Autodesk Inventor part; units mm, degrees
ref_plane "YZ Plane" through (0, 0, 0) normal (1, 0, 0) x (0, 1, 0)
ref_plane "XZ Plane" through (0, 0, 0) normal (0, 1, 0) x (-1, 0, 0)
ref_plane "XY Plane" through (0, 0, 0) normal (0, 0, 1) x (1, 0, 0)
sketch "Sketch1" plane through (0, 0, 0) normal (0, 0, 1) x (1, 0, 0)
  line L0 (-240, -100) -> (240, -100)
  line L1 (240, -100) -> (240, 100)
  line L2 (240, 100) -> (-240, 100)
  line L3 (-240, 100) -> (-240, -100)
  line L4 (-240, -100) -> (240, 100) construction
  line L5 (240, -100) -> (-240, 100) construction
  point P0 (0, 0)
  dimension "d0" = 480
  dimension "d1" = 200
extrude "Plate1" add sketch "Sketch1" along normal blind 2
sketch "Sketch2" plane through (0, 0, 0) normal (0, 0, -1) x (-1, 0, 0)
  line L0 (-220, 80) -> (-20, 80) construction
  line L1 (-20, 80) -> (-20, 60) construction
  line L2 (-20, 60) -> (-220, 60) construction
  line L3 (-220, 60) -> (-220, 80) construction
  line L4 (-240, 100) -> (240, 100)
  line L5 (-240, -100) -> (-240, 100)
  point P0 (0, 0)
  dimension "d6" = 200
  dimension "d9" = 20
  dimension "d10" = 20
  dimension "d11" = 20
mark "Mark1"
sketch "Sketch3" plane through (240, -98, 0) normal (0, -1, 0) x (1, 0, 0)
  line L0 (-480, 0) -> (0, 0)
  line L1 (0, 0) -> (0, 30)
  line L2 (0, 30) -> (-480, 30)
  line L3 (-480, 30) -> (-480, 0)
edge flange "Flange1" height 30 angle 90 thickness 2 bend radius 2.75 thickness toward (0, -1, 0) relief round relief width 2 relief depth 1 edges at (0, -100, 2) wall of the first edge with corners at (-240, -98, 0) (240, -98, 0) (240, -98, 30) (-240, -98, 30)
bend "Bend1"
corner "Corner1"
sketch "Sketch4" plane through (-240, -98, 30) normal (0, 1, 0) x (1, 0, 0)
  line L0 (480, 25.25) -> (0, 25.25)
  line L1 (0, 25.25) -> (0, 0)
  line L2 (0, 0) -> (480, 0)
  line L3 (480, 25.25) -> (480, 0)
  circle A0 centre (240, 10) radius 5
  point P0 (240, 30)
  point P1 (240, 25.25)
  point P2 (240, 0)
  dimension "d22" = 10
  dimension "d23" = 10
extrude "Cut1" cut sketch "Sketch4" against normal blind 2 contours A0
pattern_linear "Rectangular Pattern1" count 3 spacing 200 along (1, 0, 0) of "Cut1" first direction both ways yes
equation "\"d24\" = Thickness"
equation "\"d2\" = Thickness"
equation "\"d12\" = BendReliefWidth"
equation "\"d13\" = BendReliefDepth"
equation "\"d14\" = MinimumRemnant"
equation "\"d15\" = TransitionRadius"
equation "\"d18\" = BendRadius"
equation "\"d19\" = CornerReliefSize"
equation "\"d20\" = GapSize"
equation "\"d21\" = JacobiRadiusSize"
equation "\"BendReliefWidth\" = Thickness"
equation "\"BendReliefDepth\" = 0.5 * Thickness"
equation "\"CornerReliefSize\" = 4 * Thickness"
equation "\"MinimumRemnant\" = 2 * Thickness"
equation "\"TransitionRadius\" = BendRadius"
equation "\"JacobiRadiusSize\" = BendRadius"
equation "\"GapSize\" = Thickness"
properties part number "TRM 014 face main" material "AISI 304"
Read the model definition and answer for the solid it produces. Units are mm, in the model's axes. A direction names the side the tool comes from. Give positions to 0.01 mm unless a question says otherwise; leave off trailing zeros. Write each loop counter-clockwise with the first axis right and the second up, starting at its lowest first coordinate (ties: lowest second). Pieces come first, ordered by that corner, then holes. Notation, with made-up numbers: (17, 20) -> (55, 20) arc R25 ccw to (55, 34) -> close; hole circle Ø9 at (32.5, 65). An arc over 180 degrees is marked (long way). Answer as a JSON object with one key per item and string values.
1) Section D-D on y = 15 is taken. Write down the section's boundary in (x, z), then the cut area to 3 significant figures.
Findings below:
{"outline": "(-240, 0) -> (240, 0) -> (240, 2) -> (-240, 2) -> close", "area": "960 mm^2"}
2) For a pull along Z with two mould halves and no side action, classify faces 1 (the flat face through (-3, 4, 2)), 2 (the cylindrical face through (202.307, -98.986, 24.436)), 3 (the flat face through (3, -100, 15)) as pulls with the +Z half, pulls with the -Z half, needs draft (parallel to the pull), parting line crosses it, or undercut.
Findings below:
{"face 1": "pulls with the +Z half", "face 2": "undercut", "face 3": "needs draft"}
3) Straight lines are drawn through the part: probe 1 along X at (y, z) = (-98.7, 20); probe 2 along Z at (x, y) = (200, -99.05); probe 3 along Y at (x, z) = (203, 27.5). For each, find the intervals that lie inside material, in ascending order. Write a range as from..to.
Findings below:
{"probe 1": "x = -240..-205, -195..-5, 5..195, 205..240", "probe 2": "z = 1.9..15, 25..30", "probe 3": "y = -100..-98"}
4) Section B-B on z = 20 is taken. Write down the section's boundary in (x, y).
Findings below:
{"outline": "(-240, -100) -> (-205, -100) -> (-205, -98) -> (-240, -98) -> close; (-195, -100) -> (-5, -100) -> (-5, -98) -> (-195, -98) -> close; (5, -100) -> (195, -100) -> (195, -98) -> (5, -98) -> close; (205, -100) -> (240, -100) -> (240, -98) -> (205, -98) -> close"}
5) Flat-ended cylindrical pins translate along their axes: pin 1 Ø12 at (x, y) = (-95, -57) entering from -Z; pin 2 Ø1 at (x, z) = (180.5, 24) entering from +Y; pin 3 Ø8 at (x, z) = (0, 20) entering from -Y. Find the tip coordinate at first contact, or state that the pin passes through.
Findings below:
{"pin 1": "stops at z = 0", "pin 2": "stops at y = -98", "pin 3": "passes through"}
6) Section A-A on x = -200 is taken. Write down the section's boundary in (y, z), then the cut area to 3 significant figures.
Findings below:
{"outline": "(-100, 4.75) arc R4.75 ccw to (-95.25, 0) -> (100, 0) -> (100, 2) -> (-95.25, 2) arc R2.75 cw to (-98, 4.75) -> (-98, 15) -> (-100, 15) -> close; (-100, 25) -> (-98, 25) -> (-98, 30) -> (-100, 30) -> close", "area": "433 mm^2"}
7) Section C-C on x = -29.5 is taken. Write down the section's boundary in (y, z).
Findings below:
{"outline": "(-100, 4.75) arc R4.75 ccw to (-95.25, 0) -> (100, 0) -> (100, 2) -> (-95.25, 2) arc R2.75 cw to (-98, 4.75) -> (-98, 30) -> (-100, 30) -> close"}
8) A tool of negligible diameter and unlimited length cuts with its end or side. For faces 4 (the flat face through (3, -98, 14)), 5 (the cylindrical face through (-197.693, -98.986, 24.436)), from which of +Z, -Z, +X, -X, +Y, -Y can it reach the whole face along a straight path? Write none if from no direction.
Findings below:
{"face 4": "+Z, +X, -X, +Y", "face 5": "+Y, -Y"}
